Can you work these out from the model? Positions are in its coordinate system, mm. Face numbers are marked on the shaded views. A direction names the side the tool comes from. Round coordinates to 2 decimals unless told otherwise and drop trailing zeros. Order: outer loops, then holes, each group sorted by start corner. A loop starts at its lowest first (then second) coordinate and runs counter-clockwise, first axis right, second up.
Q1. For the marked faces 1, 2, 3, 4 and 5, which set-ups out of +Z, -Z, +X, -X, +Y, -Y let a thin tool reach every point of the face, with its end or its side?
Q2. If we section it at A-A (y = 11.5): Please give me the cut outline in (x, z).
Q3. If I drill on line 1 (Z direction, x = 40, y = 4.5); line 2 (Y direction, x = 55, z = -29.75); line 3 (Y direction, x = 60.5, z = -7), over which ranges is the centre line in solid material (lowest first)?
Q4. If we section it at D-D (y = 39): Please give me the cut outline in (x, z).
Q5. We'd pull the mould along X, two halves only. Please class the marked faces 6, 7, 8 and 9: pulls with the +X half, pulls with the -X half, needs draft (parallel to the pull), parting line crosses it, or undercut.
Q6. If we section it at C-C (z = -15): Please give me the cut outline in (x, y).
Q7. If we section it at B-B (x = 65.5): Please give me the cut outline in (y, z), plus the area to 3 significant figures.
Q8. Will these pins go through, and if not, where does the flat tip stop? P1, Ø1.5, axis at x = 40, z = -35.5, coming from the -Y side; P2, Ø15.5, axis at x = 17.5, z = -27.5, coming from the -Y side; P3, Ø6, axis at x = 55, y = 35, coming from the -Z side.
Autodesk Inventor part; units mm, degrees
ref_plane "YZ Plane" through (0, 0, 0) normal (1, 0, 0) x (0, 1, 0)
ref_plane "XZ Plane" through (0, 0, 0) normal (0, 1, 0) x (-1, 0, 0)
ref_plane "XY Plane" through (0, 0, 0) normal (0, 0, 1) x (1, 0, 0)
sketch "Sketch1" plane through (0, 0, 0) normal (0, 0, 1) x (1, 0, 0)
  line L0 (0, 0) -> (80, 0)
  line L1 (80, 0) -> (80, 55)
  line L2 (80, 55) -> (0, 55)
  line L3 (0, 55) -> (0, 0)
  dimension "d0" = 55
  dimension "d1" = 80
extrude "Extrusion1" add sketch "Sketch1" against normal blind 50
sketch "Sketch2" plane through (0, 0, 0) normal (0, 0, 1) x (1, 0, 0)
  line L0 (0, 0) -> (32.5, 0)
  line L1 (32.5, 0) -> (32.5, 15)
  line L2 (32.5, 15) -> (0, 15)
  line L3 (0, 15) -> (0, 0)
  line L4 (80, 55) -> (80, 0)
  line L5 (80, 0) -> (47.5, 0)
  line L6 (47.5, 0) -> (47.5, 15)
  line L7 (47.5, 15) -> (80, 15)
  line L8 (80, 15) -> (80, 0)
  dimension "d4" = 15
  dimension "d5" = 15
extrude "Extrusion2" cut sketch "Sketch2" against normal through all
sketch "Sketch3" plane through (0, 0, 0) normal (0, 0, 1) x (1, 0, 0)
  line L0 (32.5, 13.5858) -> (31.0858, 15)
  line L1 (31.0858, 15) -> (32.5, 16.4142)
  line L2 (32.5, 16.4142) -> (33.9142, 15)
  line L3 (33.9142, 15) -> (32.5, 13.5858)
  line L4 (32.5, 15) -> (32.5, 0)
  line L5 (32.5, 13.5858) -> (32.5, 16.4142) construction
  line L6 (31.0858, 15) -> (33.9142, 15) construction
  line L7 (47.5, 13.5858) -> (48.9142, 15)
  line L8 (48.9142, 15) -> (47.5, 16.4142)
  line L9 (47.5, 16.4142) -> (46.0858, 15)
  line L10 (46.0858, 15) -> (47.5, 13.5858)
  line L11 (47.5, 15) -> (80, 15)
  line L12 (47.5, 13.5858) -> (47.5, 16.4142) construction
  line L13 (48.9142, 15) -> (46.0858, 15) construction
  point P0 (0, 0)
  dimension "d8" = 2
extrude "Extrusion3" cut sketch "Sketch3" against normal through all
sketch "Sketch4" plane through (80, 55, 0) normal (1, 0, 0) x (0, 0, -1)
  line L0 (-1.4142, -20) -> (0, -18.5858)
  line L1 (0, -18.5858) -> (1.4142, -20)
  line L2 (1.4142, -20) -> (0, -21.4142)
  line L3 (0, -21.4142) -> (-1.4142, -20)
  line L4 (0, -40) -> (0, 0)
  line L5 (-1.4142, -20) -> (1.4142, -20) construction
  line L6 (0, -18.5858) -> (0, -21.4142) construction
  line L7 (0, 0) -> (50, 0)
  point P0 (0, -55)
  point P1 (0, -20)
  dimension "d11" = 2
  dimension "d12" = 20
extrude "Extrusion4" cut sketch "Sketch4" against normal through all
sketch "Sketch5" plane through (0, 55, 0) normal (0, 1, 0) x (1, 0, 0)
  line L0 (40, -1.4142) -> (38.5858, 0)
  line L1 (38.5858, 0) -> (40, 1.4142)
  line L2 (40, 1.4142) -> (41.4142, 0)
  line L3 (41.4142, 0) -> (40, -1.4142)
  line L4 (32.5, 0) -> (47.5, 0)
  line L5 (40, -1.4142) -> (40, 1.4142) construction
  line L6 (38.5858, 0) -> (41.4142, 0) construction
  point P0 (0, 0)
  point P1 (40, 0)
  dimension "d15" = 2
extrude "Extrusion5" cut sketch "Sketch5" against normal through all
sketch "Sketch6" plane through (0, 0, -50) normal (0, 0, -1) x (-1, 0, 0)
  line L0 (-55, 35) -> (-25, 35) construction
  line L1 (-41.4142, 36.4142) -> (-80, 36.4142)
  line L2 (-55, 27.5) -> (-25, 27.5)
  line L3 (-25, 42.5) -> (-55, 42.5)
  arc A0 (-55, 42.5) -> (-55, 27.5) centre (-55, 35) ccw
  arc A1 (-25, 27.5) -> (-25, 42.5) centre (-25, 35) ccw
  line L4 (0, 55) -> (-80, 55)
  line L5 (-80, 55) -> (-80, 15)
  point P0 (0, 0)
  point P1 (-40, 35)
  dimension "d18" = 7.5
  dimension "d19" = 20
  dimension "d20" = 40
  dimension "d21" = 30
extrude "Extrusion6" cut sketch "Sketch6" against normal blind 10
sketch "Sketch7" plane through (0, 0, -40) normal (0, 0, -1) x (-1, 0, 0)
  line L0 (-80, 35) -> (-40, 35)
  circle A0 centre (-40, 35) radius 7.5
  point P0 (0, 0)
  dimension "d24" = 15
extrude "Extrusion7" cut sketch "Sketch7" against normal blind 5
sketch "Sketch8" plane through (0, 0, -40) normal (0, 0, -1) x (-1, 0, 0)
  line L0 (-80, 35) -> (-40, 35)
  circle A0 centre (-55, 35) radius 2.5
  line L1 (-40, 35) -> (0, 35)
  circle A1 centre (-25, 35) radius 2.5
  point P0 (0, 0)
  dimension "d27" = 5
  dimension "d28" = 15
  dimension "d29" = 15
extrude "Extrusion8" cut sketch "Sketch8" against normal blind 18
thread "Thread1"
thread "Thread2"
chamfer "Chamfer1" distance 0.75 angle 45 5 edges at (40, 55, -50) (80, 55, -25) (0, 55, -25) (0, 35, -50) (80, 35, -50)
sketch "Sketch9" plane through (32.5, 0, -50) normal (0, -1, 0) x (1, 0, 0)
  circle A0 centre (7.5, 35) radius 2.5
  circle A1 centre (7.5, 15) radius 2.5
  line L0 (15, 0) -> (0, 0)
  point P0 (-32.5, 50)
  point P1 (7.5, 48.5858)
  dimension "d39" = 5
  dimension "d40" = 20
  dimension "d41" = 15
extrude "Extrusion9" cut sketch "Sketch9" against normal blind 18
thread "Thread3"
thread "Thread4"
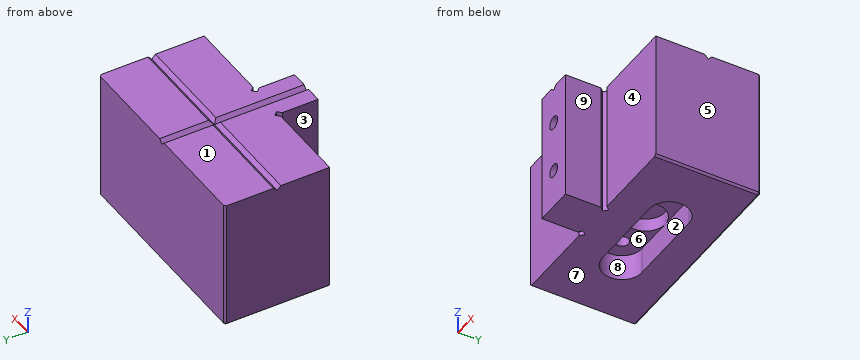
Solution:
1. face 1: +Z, +X, -X, +Y, -Y
1. face 2: -Z
1. face 3: +Z, -Z, -X, -Y
1. face 4: +Z, -Z, +X, -Y
1. face 5: +Z, -Z, +X, +Y, -Y
2. outline: (32.5, -50) - (47.5, -50) - (47.5, 0) - (41.41, 0) - (40, -1.41) - (38.59, 0) - (32.5, 0) - close; hole circle Ø5 at (40, -35); hole circle Ø5 at (40, -15)
3. line 1: z = -50 to -37.5, -32.5 to -17.5, -12.5 to -1.41
3. line 2: y = 15 to 32.5, 37.5 to 55
3. line 3: y = 15 to 55
4. outline: (0, -49.25) - (0.75, -50) - (18.66, -50) - (18.66, -40) - (33.66, -40) - (33.66, -35) - (46.34, -35) - (46.34, -40) - (61.34, -40) - (61.34, -50) - (79.25, -50) - (80, -49.25) - (80, 0) - (41.41, 0) - (40, -1.41) - (38.59, 0) - (0, 0) - close
5. face 6: undercut
5. face 7: needs draft
5. face 8: undercut
5. face 9: pulls with the +X half
6. outline: (0, 15) - (31.09, 15) - (32.5, 16.41) - (33.91, 15) - (32.5, 13.59) - (32.5, 0) - (37.5, 0) - (37.5, 18) - (42.5, 18) - (42.5, 0) - (47.5, 0) - (47.5, 13.59) - (46.09, 15) - (47.5, 16.41) - (48.91, 15) - (80, 15) - (80, 54.25) - (79.25, 55) - (0.75, 55) - (0, 54.25) - close
7. outline: (15, -50) - (54.25, -50) - (55, -49.25) - (55, 0) - (36.41, 0) - (35, -1.41) - (33.59, 0) - (15, 0) - close
7. area: 2,000 mm2
8. P1: stops at y = 18
8. P2: stops at y = 15
8. P3: stops at z = -40
